Can you work these out from the model? Positions are in its coordinate system, mm. Coordinates: 2 decimals unless noted, no trailing zeros. Write each loop counter-clockwise with the first axis right and the second up, starting at its lowest first coordinate (ties: lowest second). Pieces come first, ordered by that corner, then holes. Notation, with made-up numbers: (50.5, -14.75) -> (55.5, -14.75) arc R9 cw to (55.5, 2.25) -> close; hole circle Ø10 at (55, 20.5). An arc over 180 degrees is marked (long way). Use one line per item in the form item = value.
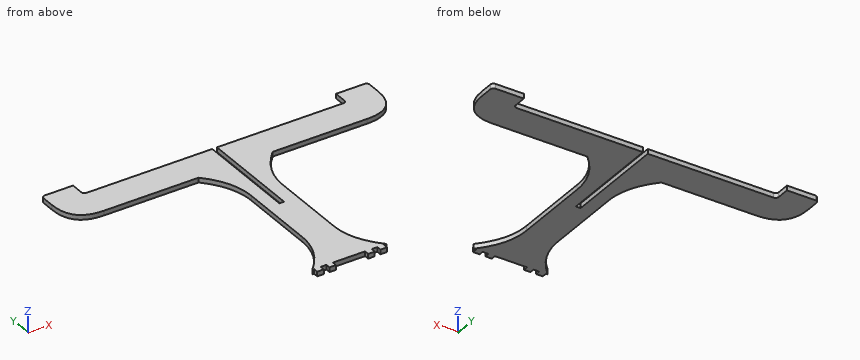
```python
from build123d import *

# Parameters (mm, degrees)
P_IDAT_VYSUNUT_M2_DEPTH  = 3
SKICA2_W                 = 3
SKICA2_H                 = 65
ODEBRAT_VYSUNUT_M3_DEPTH = 3


with BuildPart() as part:
    # Skica1 → Přidat vysunutím2 (new body)
    with BuildSketch(Plane.XY):
        with BuildLine():
            Line((-90.642636358, 2.694256757), (-30.642636358, 2.694256757))
            add(Edge.make_bspline(
                [(-30.642636358, 2.694256757), (-17.025139471, -11.118063286), (-17.142636358, -27.878389443)],
                knots=[0, 0, 0, 1, 1, 1], degree=2))
            Line((-17.142636358, -27.878389443), (-17.142636358, -76.655981804))
            add(Edge.make_bspline(
                [(-30.642636358, -107.305743243), (-17.009316786, -93.458261678), (-17.142636358, -76.655981804)],
                knots=[0, 0, 0, 1, 1, 1], degree=2))
            Line((-30.642636358, -107.305743243), (-29.497972973, -107.305743243))
            Line((-29.497972973, -107.305743243), (-29.497972973, -110.305743243))
            Line((-29.497972973, -110.305743243), (-25.347972973, -110.305743243))
            Line((-25.347972973, -110.305743243), (-25.347972973, -107.305743243))
            Line((-25.347972973, -107.305743243), (-21.697972973, -107.305743243))
            Line((-21.697972973, -107.305743243), (-21.697972973, -110.305743243))
            Line((-21.697972973, -110.305743243), (-17.547972973, -110.305743243))
            Line((-17.547972973, -110.305743243), (-17.547972973, -107.305743243))
            Line((-17.547972973, -107.305743243), (2.852027027, -107.305743243))
            Line((2.852027027, -107.305743243), (2.852027027, -110.305743243))
            Line((2.852027027, -110.305743243), (7.002027027, -110.305743243))
            Line((7.002027027, -110.305743243), (7.002027027, -107.305743243))
            Line((7.002027027, -107.305743243), (10.652027027, -107.305743243))
            Line((10.652027027, -107.305743243), (10.652027027, -110.305743243))
            Line((10.652027027, -110.305743243), (14.802027027, -110.305743243))
            Line((14.802027027, -110.305743243), (14.802027027, -107.305743243))
            Line((14.802027027, -107.305743243), (16.357363642, -107.305743243))
            add(Edge.make_bspline(
                [(16.357363642, -107.305743243), (2.72404407, -93.458261678), (2.857363642, -76.655981804)],
                knots=[0, 0, 0, 1, 1, 1], degree=2))
            Line((2.857363642, -76.655981804), (2.857363642, -27.878389443))
            add(Edge.make_bspline(
                [(16.357363642, 2.694256757), (2.739866756, -11.118063286), (2.857363642, -27.878389443)],
                knots=[0, 0, 0, 1, 1, 1], degree=2))
            Line((16.357363642, 2.694256757), (76.357363642, 2.694256757))
            add(Edge.make_bspline(
                [(96.357363642, 22.694256757), (96.357363642, 2.694256757), (76.357363642, 2.694256757)],
                knots=[0, 0, 0, 1, 1, 1], degree=2))
            Line((96.357363642, 22.694256757), (96.357363642, 30.694256757))
            ThreePointArc((96.357363642, 30.694256757), (95.771577204, 32.108470319), (94.357363642, 32.694256757))
            Line((94.357363642, 32.694256757), (76.357363642, 32.694256757))
            Line((76.357363642, 32.694256757), (76.357363642, 24.694256757))
            ThreePointArc((76.357363642, 24.694256757), (75.771577204, 23.280043194), (74.357363642, 22.694256757))
            Line((74.357363642, 22.694256757), (-88.642636358, 22.694256757))
            ThreePointArc((-88.642636358, 22.694256757), (-90.05684992, 23.280043194), (-90.642636358, 24.694256757))
            Line((-90.642636358, 24.694256757), (-90.642636358, 32.694256757))
            Line((-90.642636358, 32.694256757), (-108.642636358, 32.694256757))
            ThreePointArc((-108.642636358, 32.694256757), (-110.05684992, 32.108470319), (-110.642636358, 30.694256757))
            Line((-110.642636358, 30.694256757), (-110.642636358, 22.694256757))
            add(Edge.make_bspline(
                [(-110.642636358, 22.694256757), (-110.642636358, 2.694256757), (-90.642636358, 2.694256757)],
                knots=[0, 0, 0, 1, 1, 1], degree=2))
        make_face()
    extrude(amount=P_IDAT_VYSUNUT_M2_DEPTH)

    # Skica2 → Odebrat vysunutím3 (cut)
    with BuildSketch(Plane(origin=(0, 0, 0), x_dir=(-1, 0, 0), z_dir=(0, 0, -1))):
        with Locations((7.347972973, -9.805743243)):
            Rectangle(SKICA2_W, SKICA2_H)
    extrude(amount=-ODEBRAT_VYSUNUT_M3_DEPTH, mode=Mode.SUBTRACT)


solid = part.part
```
Q1. Suppose I cut it at A-A (y = -38). Write out the boundary of the cut face in (x, z).
Return value:
outline = (-17.14, 0) -> (-8.85, 0) -> (-8.85, 3) -> (-17.14, 3) -> close; (-5.85, 0) -> (2.86, 0) -> (2.86, 3) -> (-5.85, 3) -> close
Q2. If I drill on line 1 (X direction, y = -39, z = 1.35); line 2 (X direction, y = 26, z = 0.5); line 3 (Y direction, x = -13, z = 1.3), over which ranges is the centre line in solid material (lowest first)? Write a range as from..to.
Return value:
line_1 = -17.14..-8.85, -5.85..2.86
line_2 = -110.64..-90.64, 76.36..96.36
line_3 = -107.31..22.69
Q3. Will these pins go through, and if not, where does the flat tip stop? pin 1 (0.9 mm diameter, centred on y = -108.5, z = 2, fed in from +X); pin 2 (1.2 mm diameter, centred on x = 15.5, z = 1.5, fed in from -Y); pin 3 (0.9 mm diameter, centred on y = -109.5, z = 2, fed in from -X).
Return value:
pin_1 = 14.8
pin_2 = -107.31
pin_3 = -29.5
Q4. Suppose I cut it at B-B (x = 55.5). Write out the boundary of the cut face in (y, z), then the cut area to 3 significant figures.
Return value:
outline = (2.69, 0) -> (22.69, 0) -> (22.69, 3) -> (2.69, 3) -> close
area = 60.0 mm2
